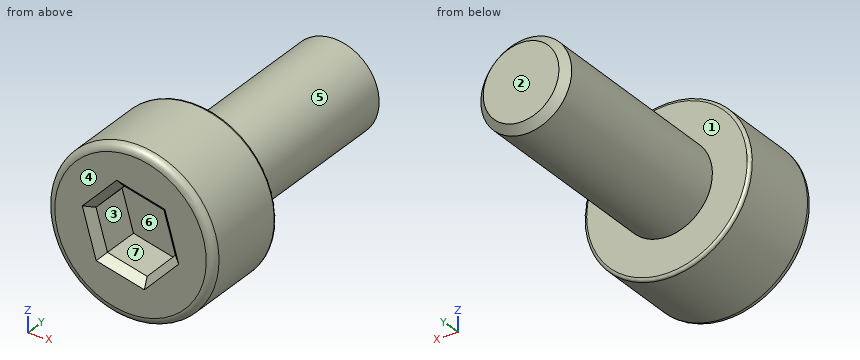
```python
from build123d import *

# Parameters (mm, degrees)
SKETCH1_R           = 2.75
BOSS_EXTRUDE1_DEPTH = 3
SKETCH2_R           = 1.5
BOSS_EXTRUDE2_DEPTH = 7
CUT_EXTRUDE1_DEPTH  = 1.5
CHAMFER1_SIZE       = 0.25
FILLET1_R           = 0.25
CHAMFER2_SIZE       = 0.25
FILLET2_R           = 0.1


with BuildPart() as part:
    # Sketch1 → Boss-Extrude1 (new body)
    with BuildSketch(Plane(origin=(0, 0, 0), x_dir=(1, 0, 0), z_dir=(0, 1, 0))):
        with Locations(Location((0, 0, 0), (0, 0, 270))):
            Circle(SKETCH1_R)
    extrude(amount=BOSS_EXTRUDE1_DEPTH)

    # Sketch2 → Boss-Extrude2 (add)
    with BuildSketch(Plane(origin=(0, 3, 0), x_dir=(1, 0, 0), z_dir=(0, 1, 0))):
        with Locations(Location((0, 0, 0), (0, 0, 270))):
            Circle(SKETCH2_R)
    extrude(amount=BOSS_EXTRUDE2_DEPTH)

    # Sketch3 → Cut-Extrude1 (cut)
    with BuildSketch(Plane.XZ):
        Polygon((0.934168857, 0.974591477), (-0.376936549, 1.2963097), (-1.311105406, 0.321718223), (-0.934168857, -0.974591477), (0.376936549, -1.2963097), (1.311105406, -0.321718223), align=None)
    extrude(amount=-CUT_EXTRUDE1_DEPTH, mode=Mode.SUBTRACT)

    # Chamfer1
    chamfer1_edges = [part.edges().sort_by_distance(p)[0] for p in [
        (1.122637131, 0, 0.326436627),
        (0.278616154, 0, 1.135450588),
        (-0.844020977, 0, 0.809013962),
        (-1.122637131, 0, -0.326436627),
        (-0.278616154, 0, -1.135450588),
        (0.844020977, 0, -0.809013962),
    ]]
    chamfer(chamfer1_edges, length=CHAMFER1_SIZE)

    # Fillet1
    fillet1_edges = [part.edges().sort_by_distance(p)[0] for p in [
        (0, 0, -2.75),
    ]]
    fillet(fillet1_edges, radius=FILLET1_R)

    # Chamfer2
    chamfer2_edges = [part.edges().sort_by_distance(p)[0] for p in [
        (0, 10, -1.5),
    ]]
    chamfer(chamfer2_edges, length=CHAMFER2_SIZE)

    # Fillet2
    fillet2_edges = [part.edges().sort_by_distance(p)[0] for p in [
        (0, 3, -2.75),
    ]]
    fillet(fillet2_edges, radius=FILLET2_R)


solid = part.part
```
Design review of the part built by this model. Coordinates are the model's own, in mm. Face numbers are marked on the shaded views. A direction names the side the tool comes from. Coordinates: 2 decimals unless noted, no trailing zeros. Order: outer loops, then holes, each group sorted by start corner. A loop starts at its lowest first (then second) coordinate and runs counter-clockwise, first axis right, second up.
1) Mouldability with a two-part tool opening along X and no side actions: class the marked faces 4, 5, 6 and 7 as +X half, -X half, draft (parallel to the pull), parting line (faces both ways), or undercut.
2) Take a section at C-C, the plane y = 6.75. Give the boundary of the cut face in (x, z).
3) For the marked faces 1, 2 and 3, list the 3-axis set-ups (+Z, -Z, +X, -X, +Y, -Y) from which the entire face can be reached by the end or side of a thin tool; tool diameter is ignored.
4) Take a section at A-A, the plane x = 0. Give the boundary of the cut face in (y, z), and give its area (3 significant figures).
5) Wall thickness on line 1 along Y through (x, z) = (1.4, -1); line 2 along X through (y, z) = (1.75, 0.1); line 3 along Z through (x, y) = (0.5, 0.75): over which ranges is each line inside the solid? List them lowest first.
6) Take a section at B-B, the plane z = 0. Give the boundary of the cut face in (x, y).
Returned:
1. face 4: draft
1. face 5: parting line
1. face 6: undercut
1. face 7: undercut
2. outline: circle Ø3 at (0, 0)
3. face 1: +Y
3. face 2: +Z, -Z, +X, -X, +Y
3. face 3: -Y
4. outline: (0, -2.5) arc R0.25 ccw to (0.25, -2.75) - (2.9, -2.75) arc R0.1 ccw to (3, -2.65) - (3, -1.5) - (9.75, -1.5) - (10, -1.25) - (10, 1.25) - (9.75, 1.5) - (3, 1.5) - (3, 2.65) arc R0.1 ccw to (2.9, 2.75) - (0.25, 2.75) arc R0.25 ccw to (0, 2.5) - (0, 1.46) - (0.25, 1.2) - (1.5, 1.2) - (1.5, -1.2) - (0.25, -1.2) - (0, -1.46) - close
4. area: 33.7 mm2
5. line 1: y = 0 to 3
5. line 2: x = -2.75 to 2.75
5. line 3: z = -2.7 to -1.17, 1.08 to 2.7
6. outline: (-2.75, 0.25) arc R0.25 ccw to (-2.5, 0) - (-1.48, 0) - (-1.22, 0.25) - (-1.22, 1.5) - (1.22, 1.5) - (1.22, 0.25) - (1.48, 0) - (2.5, 0) arc R0.25 ccw to (2.75, 0.25) - (2.75, 2.9) arc R0.1 ccw to (2.65, 3) - (1.5, 3) - (1.5, 9.75) - (1.25, 10) - (-1.25, 10) - (-1.5, 9.75) - (-1.5, 3) - (-2.65, 3) arc R0.1 ccw to (-2.75, 2.9) - close
